from build123d import *

# Parameters (mm, degrees)
F0_W     = 76.2
F0_H     = 76.2
F1_DEPTH = 76.2
F2_W     = 57.15
F2_H     = 57.15
F3_DEPTH = 57.15
F4_R     = 12.7
F5_DEPTH = 19.05
F6_R     = 12.7
F7_DEPTH = 19.05
F8_R     = 12.7
F9_DEPTH = 19.05
F10_SIZE = 6.35
F11_R    = 6.35


with BuildPart() as f1:
    # F0 (on Front) → F1 (new body)
    with BuildSketch(Plane.XZ):
        with Locations((38.1, 38.1)):
            Rectangle(F0_W, F0_H)
    extrude(amount=F1_DEPTH)

    # F2 (on face) → F3 (cut)
    with BuildSketch(Plane.XZ.offset(76.2)):
        with Locations((47.625, 47.625)):
            Rectangle(F2_W, F2_H)
    extrude(amount=-F3_DEPTH, mode=Mode.SUBTRACT)

    # F4 (on face) → F5 (cut)
    with BuildSketch(Plane.XY.offset(19.05)):
        with Locations((47.625, -47.625)):
            Circle(F4_R)
    extrude(amount=-F5_DEPTH, mode=Mode.SUBTRACT)

    # F6 (on face) → F7 (cut)
    with BuildSketch(Plane.YZ.offset(19.05)):
        with Locations((-47.625, 47.625)):
            Circle(F6_R)
    extrude(amount=-F7_DEPTH, mode=Mode.SUBTRACT)

    # F8 (on face) → F9 (cut)
    with BuildSketch(Plane.XZ.offset(19.05)):
        with Locations((47.625, 47.625)):
            Circle(F8_R)
    extrude(amount=-F9_DEPTH, mode=Mode.SUBTRACT)

    # F10
    f10_edges = [f1.edges().sort_by_distance(p)[0] for p in [
        (9.525, -76.2, 76.2),
        (76.2, -9.525, 76.2),
    ]]
    chamfer(f10_edges, length=F10_SIZE)

    # F11
    f11_edges = [f1.edges().sort_by_distance(p)[0] for p in [
        (19.05, -19.05, 47.625),
    ]]
    fillet(f11_edges, radius=F11_R)


solid = f1.part
For this review, take the finished solid that the model builds, in its own axes (mm). A direction names the side the tool comes from. Give positions to 0.01 mm unless a question says otherwise; leave off trailing zeros. Order: outer loops, then holes, each group sorted by start corner. A loop starts at its lowest first (then second) coordinate and runs counter-clockwise, first axis right, second up. Notation, with made-up numbers: M 25.5,35 L 66.5,35 A27 cw 66.5,70 Z; hole C 40.5,5.25 d4. An arc over 180 degrees is marked long. Answer in a Markdown table with one row per item. Add a question column.
(1) Consider section D-D on x = 43. State the section outline as (y, z) points.
(2) Mouldability with a two-part tool opening along X and no side actions: class faces 3 (the face through (59.74, -9.66, 51.44)), 4 (the face through (19.05, -62, 47)), 5 (the face through (26.7, -18.9, 76.2)) as +X half, -X half, draft (parallel to the pull), parting line (faces both ways), or undercut.
(3) Consider section B-B on y = -46. State the section outline as (x, z) points.
(4) For faces 1 (the face through (20.86, -20.96, 48.03)), 2 (the face through (9.39, -72.98, 73.07)), list the 3-axis set-ups (+Z, -Z, +X, -X, +Y, -Y) from which the entire face can be reached by the end or side of a thin tool; tool diameter is ignored.
(5) Wall thickness on probe 1 along X at (y, z) = (-66.5, 25); probe 2 along Y at (x, z) = (36.5, 39.5): over which ranges is each line inside the solid? List them lowest first. Write a range as [from, to].
(6) Consider section C-C on z = 37.5. State the section outline as (x, y) points.
(7) Consider section A-A on z = 64. State the section outline as (x, y) points, and give its area (3 significant figures).
(8) For pin 1 (8 mm diameter, centred on y = -27, z = 36.5, fed in from +X); pin 2 (12 mm diameter, centred on x = 30, z = 51, fed in from -Y); pin 3 (1.5 mm diameter, centred on y = -58, z = 66.5, fed in from +X); pin 4 (6 mm diameter, centred on x = 22, y = -44, fed in from -Z), all flat-tipped, find the tip position at first contact; note any pin that passes through.
Evaluation:
| question | item | result |
|---|---|---|
| 1 | outline | M -76.2,0 L -59.45,0 L -59.45,19.05 L -76.2,19.05 Z; M -35.8,0 L 0,0 L 0,35.8 L -19.05,35.8 L -19.05,19.05 L -35.8,19.05 Z; M -19.05,59.45 L 0,59.45 L 0,76.2 L -19.05,76.2 Z |
| 2 | face 3 | undercut |
| 2 | face 4 | +X half |
| 2 | face 5 | draft |
| 3 | outline | M 0,0 L 35.03,0 L 35.03,19.05 L 19.05,19.05 L 19.05,35.03 L 0,35.03 Z; M 0,60.22 L 19.05,60.22 L 19.05,76.2 L 0,76.2 Z; M 60.22,0 L 76.2,0 L 76.2,19.05 L 60.22,19.05 Z |
| 4 | face 1 | +Z, +X, -Y |
| 4 | face 2 | +Z, +X, -X, -Y |
| 5 | probe 1 | x = [0, 19.05] |
| 5 | probe 2 | y = [-19.05, 0] |
| 6 | outline | M 0,-76.2 L 19.05,-76.2 L 19.05,-55.29 L 0,-55.29 Z; M 0,-39.96 L 19.05,-39.96 L 19.05,-25.4 A6.35 cw 25.4,-19.05 L 39.96,-19.05 L 39.96,0 L 0,0 Z; M 55.29,-19.05 L 76.2,-19.05 L 76.2,0 L 55.29,0 Z |
| 7 | outline | M 0,-76.2 L 19.05,-76.2 L 19.05,-25.4 A6.35 cw 25.4,-19.05 L 76.2,-19.05 L 76.2,0 L 0,0 Z |
| 7 | area | 2,550 mm^2 |
| 8 | pin 1 | stops at x = 19.52 |
| 8 | pin 2 | stops at y = -19.21 |
| 8 | pin 3 | stops at x = 19.05 |
| 8 | pin 4 | stops at z = 0 |
